Can you work these out from the drawing? Everything is in mm from the part's minimum corner. A direction names the side the tool comes from. Round coordinates to 2 decimals unless told otherwise and drop trailing zeros. Write each loop counter-clockwise with the first axis right and the second up, starting at its lowest first coordinate (ties: lowest second). Pieces come first, ordered by that corner, then holes. Notation, with made-up numbers: M 51.25,23 L 105.25,23 A7 ccw 105.25,27 Z; hole C 6,85.5 d2. An arc over 180 degrees is marked long. Answer in a Markdown table with one row per item. Add a question column.
(1) Suppose I cut it at B-B, the plane x = 30. Write out the boundary of the cut face in (y, z).
(2) I'm going to push flat-ended pins straight in: pin 1 (2 mm diameter, centred on y = 45, z = 113.5, fed in from -X) (1 decimal); pin 2 (12 mm diameter, centred on x = 25, z = 129, fed in from +Y); pin 3 (1 mm diameter, centred on x = 8, y = 23, fed in from -Z). Where does each tip first touch, or does it pass through?
(3) If I drill on probe 1 along Z at (x, y) = (33, 30); probe 2 along Z at (x, y) = (47, 12); probe 3 along Y at (x, z) = (29.5, 112.5), over which ranges is the centre line in solid material (lowest first)?
(4) For the marked faces 1 and 2, which set-ups out of +Z, -Z, +X, -X, +Y, -Y let a thin tool reach every point of the face, with its end or its side?
(5) Suppose I cut it at C-C, the plane z = 91. Write out the boundary of the cut face in (x, y).
(6) Suppose I cut it at A-A, the plane y = 30. Write out the boundary of the cut face in (x, z).
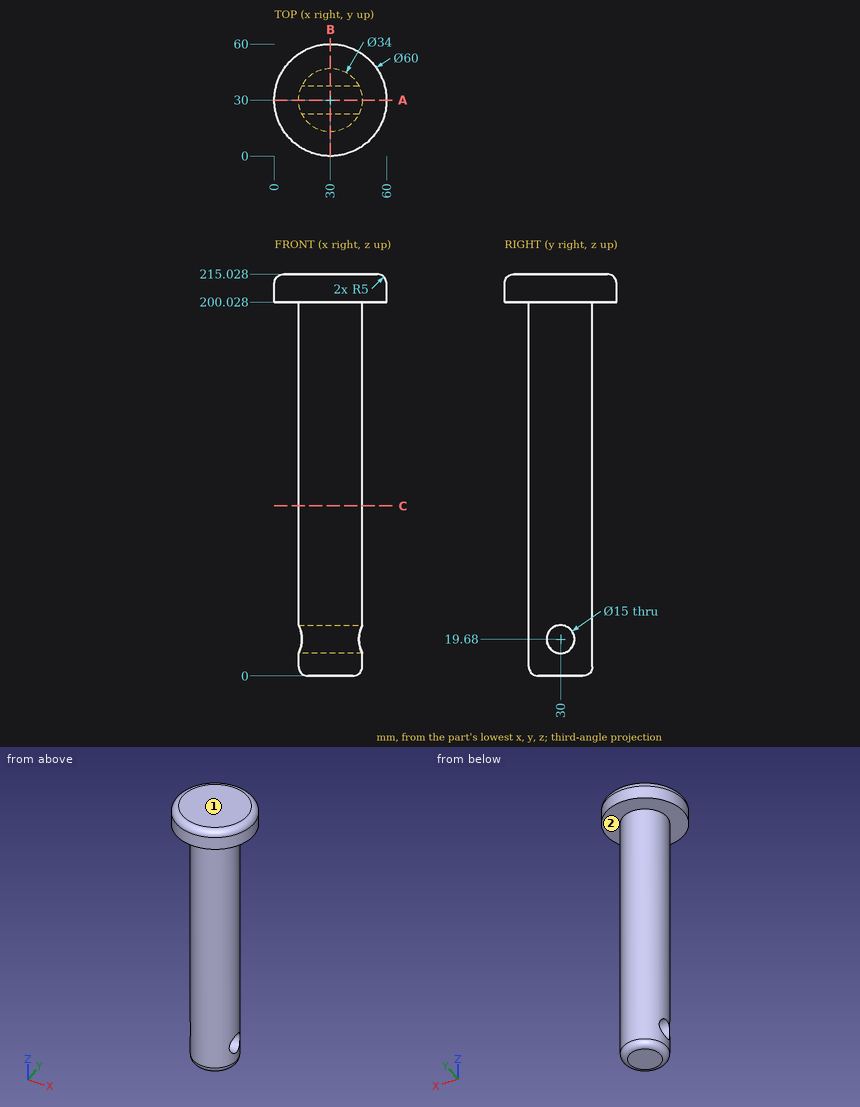
Calculated:
| question | item | result |
|---|---|---|
| 1 | outline | M 0,200.03 L 13,200.03 L 13,5 A5 ccw 18,0 L 42,0 A5 ccw 47,5 L 47,200.03 L 60,200.03 L 60,210.03 A5 ccw 55,215.03 L 5,215.03 A5 ccw 0,210.03 Z; hole C 30,19.68 d15 |
| 2 | pin 1 | x = 20.4 |
| 2 | pin 2 | y = 47 |
| 2 | pin 3 | z = 200.03 |
| 3 | probe 1 | 0 to 12.18, 27.18 to 215.03 |
| 3 | probe 2 | 200.03 to 215.03 |
| 3 | probe 3 | 13.01 to 46.99 |
| 4 | face 1 | +Z, +X, -X, +Y, -Y |
| 4 | face 2 | -Z |
| 5 | outline | C 30,30 d34 |
| 6 | outline | M 0,200.03 L 13,200.03 L 13,27.18 L 47,27.18 L 47,200.03 L 60,200.03 L 60,210.03 A5 ccw 55,215.03 L 5,215.03 A5 ccw 0,210.03 Z; M 13,5 A5 ccw 18,0 L 42,0 A5 ccw 47,5 L 47,12.18 L 13,12.18 Z |
